Source: CAD feature listing. Evaluate the final solid. Frame: model axes, mm. A direction names the side the tool comes from. Coordinates: 2 decimals unless noted, no trailing zeros. Write each loop counter-clockwise with the first axis right and the second up, starting at its lowest first coordinate (ties: lowest second). Pieces come first, ordered by that corner, then holes. Notation, with made-up numbers: (5.25, 29) -> (27.25, 29) arc R17 ccw to (27.25, 35) -> close; hole circle Ø4 at (30, 36.25). An arc over 180 degrees is marked (long way). Write item = value, one per line.
Autodesk Inventor part; units mm, degrees
ref_plane "YZ Plane" through (0, 0, 0) normal (1, 0, 0) x (0, 1, 0)
ref_plane "XZ Plane" through (0, 0, 0) normal (0, 1, 0) x (-1, 0, 0)
ref_plane "XY Plane" through (0, 0, 0) normal (0, 0, 1) x (1, 0, 0)
sketch "Sketch1" plane through (0, 0, 0) normal (0, 0, 1) x (1, 0, 0)
  line L0 (-4.4, 10.85) -> (4.4, 10.85)
  line L1 (4.4, 10.85) -> (4.4, 0)
  line L2 (4.4, 0) -> (-4.4, 0)
  line L3 (-4.4, 0) -> (-4.4, 10.85)
  point P0 (0, 0)
  dimension "d0" = 8.8
  dimension "d1" = 4.4
  dimension "d2" = 0
  dimension "d3" = 10.85
extrude "Extrusion1" add sketch "Sketch1" against normal blind 3.4
sketch "Sketch2" plane through (0, 0, -3.4) normal (0, 0, -1) x (-1, 0, 0)
  line L0 (-4.4, 10.85) -> (-4.4, 0)
  line L1 (-4.4, 6.45) -> (-4.4, 5.425)
  line L2 (4.4, 10.85) -> (-4.4, 10.85)
  line L3 (4.4, 0) -> (4.4, 10.85)
  line L4 (4.4, 6.45) -> (4.4, 4.887)
  arc A0 (4.4, 6.45) -> (-4.4, 6.45) centre (0, 6.45) ccw
  line L5 (-4.4, 0) -> (4.4, 0)
  line L6 (-4.4, 5.425) -> (-4.4, 0)
  line L7 (-4.4, 0) -> (4.4, 0)
  line L8 (4.4, 0) -> (4.4, 4.887)
  point P0 (0, 0)
extrude "Extrusion2" add sketch "Sketch2" along normal blind 10.1 contours A0 L3 L5 L0
sketch "Sketch3" plane through (0, 0, 0) normal (0, 0, 1) x (1, 0, 0)
  circle A0 centre (0, 6.5) radius 2.5
  line L0 (-4.4, 10.85) -> (4.4, 10.85)
  point P0 (0, 0)
  dimension "d8" = 4.35
  dimension "d9" = 5
extrude "Extrusion3" cut sketch "Sketch3" against normal blind 8
sketch "Sketch4" plane through (-4.4, 0, 0) normal (0, -1, 0) x (1, 0, 0)
  line L0 (8.8, -3.4) -> (8.8, -13.5)
  line L1 (8.8, -9.6102) -> (8.8, -6.6102)
  line L2 (0, -13.5) -> (8.8, -13.5)
  line L3 (5.9, -13.5) -> (2.9, -13.5)
  line L4 (2.9, -13.5) -> (2.9, -13.2)
  line L5 (2.9, -13.2) -> (5.9, -13.2)
  line L6 (5.9, -13.2) -> (5.9, -13.5)
  line L7 (8.5, -12.24) -> (8.8, -12.24)
  line L8 (8.8, -12.24) -> (8.8, -9.24)
  line L9 (8.8, -9.24) -> (8.5, -9.24)
  line L10 (8.5, -9.24) -> (8.5, -12.24)
  line L11 (2.9, -7.49) -> (5.9, -7.49)
  line L12 (5.9, -7.49) -> (5.9, -7.74)
  line L13 (5.9, -7.74) -> (2.9, -7.74)
  line L14 (2.9, -7.74) -> (2.9, -7.49)
  line L15 (8.8, 0) -> (0, 0)
  point P0 (4.4, 0)
  dimension "d12" = 3
  dimension "d14" = 3
  dimension "d15" = 1.5
  dimension "d16" = 3
  dimension "d17" = 1.5
  dimension "d18" = 0.3
  dimension "d19" = 0.25
  dimension "d20" = 0.3
  dimension "d22" = 9.24
  dimension "d24" = 7.49
  dimension "d28" = 0
extrude "Extrusion4" add sketch "Sketch4" along normal blind 4.3
fillet "Fillet1" radius 1.5 6 edges at (4.25, -4.3, -9.24) (4.25, -4.3, -12.24) (-1.5, -4.3, -7.615) (1.5, -4.3, -7.615) (-1.5, -4.3, -13.35) (1.5, -4.3, -13.35)
sketch "Sketch5" plane through (0, 6.5, -8) normal (0, 0, 1) x (1, 0, 0)
  circle A0 centre (0, 0) radius 1
  point P0 (0, -6.5)
  dimension "d29" = 2
extrude "Extrusion5" add sketch "Sketch5" along normal blind 7
fillet "Fillet2" radius 1 1 edges at (-1, 6.5, -1)
properties part number "5mm_BarrelJack"
1) First-contact query: pin 1 Ø0.9 at (x, y) = (0.5, -1.5) entering from +Z; pin 2 Ø3.5 at (y, z) = (-2, -11.5) entering from -X. Flat tips, straight axial feed; report the tip coordinate or a pass-through.
Answer block:
pin_1 = -7.49
pin_2 = -1.5
2) Cut plane B-B, the plane x = -1.25. Output: boundary loops of the cut face in (y, z), and give its area (3 significant figures).
Answer block:
outline = (-3.63, -13.5) -> (10.67, -13.5) -> (10.67, -3.4) -> (10.85, -3.4) -> (10.85, 0) -> (8.67, 0) -> (8.67, -8) -> (4.33, -8) -> (4.33, 0) -> (0, 0) -> (0, -7.49) -> (-3.63, -7.49) -> (-3.63, -7.74) -> (0, -7.74) -> (0, -13.2) -> (-3.63, -13.2) -> close
area = 112 mm2
3) Cut plane A-A, the plane z = -2.25. Output: boundary loops of the cut face in (x, y).
Answer block:
outline = (-4.4, 0) -> (4.4, 0) -> (4.4, 10.85) -> (-4.4, 10.85) -> close; circle Ø2 at (0, 6.5); hole circle Ø5 at (0, 6.5)
4) Reachability of faces 1 (the flat face through (3, 10, -3.4)), 2 (the flat face through (0, 5, -8)), 3 (the cylindrical face through (0.1, 10.85, -8.38)) from +Z, -Z, +X, -X, +Y, -Y: full face, straight path, thin tool, end or side. Return the list, or none.
Answer block:
face_1 = -Z, +X, +Y
face_2 = +Z
face_3 = -Z, +Y
5) Cut plane C-C, the plane z = -8.25. Output: boundary loops of the cut face in (x, y).
Answer block:
outline = (-4.4, 0) -> (4.4, 0) -> (4.4, 6.45) arc R4.4 ccw to (-4.4, 6.45) -> close
6) Material intervals for probe 1 along Y at (x, z) = (0, -5.5); probe 2 along Z at (x, y) = (1.25, -3.25); probe 3 along Y at (x, z) = (-0.75, -4.5), sorted ascending. Write a range as [from, to].
Answer block:
probe_1 = [0, 4], [5.5, 7.5], [9, 10.85]
probe_2 = [-13.5, -13.2], [-7.74, -7.49]
probe_3 = [0, 4.12], [5.84, 7.16], [8.88, 10.79]
7) Pull-direction query (Z, two-part tool) for faces 4 (the cylindrical face through (4.25, -3.87, -11.79)), 5 (the cylindrical face through (-0.13, 5.51, -5.04)), 6 (the flat face through (0, -2, -13.2)), 7 (the cylindrical face through (4.25, -3.87, -9.69)); classes: +Z half, -Z half, draft (parallel to the pull), parting line (faces both ways), or undercut.
Answer block:
face_4 = -Z half
face_5 = draft
face_6 = undercut
face_7 = +Z half
8) Cut plane D-D, the plane x = 2.25. Output: boundary loops of the cut face in (y, z).
Answer block:
outline = (0, -13.5) -> (10.23, -13.5) -> (10.23, -3.4) -> (10.85, -3.4) -> (10.85, 0) -> (7.59, 0) -> (7.59, -8) -> (5.41, -8) -> (5.41, 0) -> (0, 0) -> close
